```python
from build123d import *

# Parameters (mm, degrees)
CUT_EXTRUDE1_SOCKET_SLIT_DEPTH  = 18.588952107
CIRPATTERN1_PATTERN_SLITS_COUNT = 4
CHAMFER1_SIZE                   = 0.762
FILLET1_R                       = 0.762


with BuildPart() as part:
    # Sketch1 → Revolve1 - main body (revolve)
    with BuildSketch(Plane.XY):
        with BuildLine():
            Line((0, 0), (0, 13.751471687))
            ThreePointArc((0, 13.751471687), (-4.410161159, 16.183513693), (-4.70662, 21.211083874))
            Line((-4.70662, 21.211083874), (-6.08215434, 21.867194596))
            Line((-6.08215434, 21.867194596), (-7.191504241, 21.867194596))
            ThreePointArc((-7.191504241, 21.867194596), (-7.193470164, 16.069866844), (-3.175, 11.891241417))
            Line((-3.175, 11.891241417), (-3.175, 9.351241417))
            ThreePointArc((-3.175, 9.351241417), (-4.937771284, 3.538112772), (0, 0))
        make_face()
    revolve(axis=Axis((0, 0, 0), (0, -1, 0)))

    # Sketch2 → Cut-Extrude1 - socket slit (cut, through all)
    with BuildSketch(Plane(origin=(0, 13.751471687, 0), x_dir=(-1, 0, 0), z_dir=(0, -1, 0))):
        with BuildLine():
            Line((0, 0.254), (9.731504241, 0.254))
            ThreePointArc((9.731504241, 0.254), (9.985504241, 0), (9.731504241, -0.254))
            Line((9.731504241, -0.254), (0, -0.254))
            ThreePointArc((0, -0.254), (-0.254, 0), (0, 0.254))
        make_face()
    cut_extrude1_socket_slit = extrude(amount=-CUT_EXTRUDE1_SOCKET_SLIT_DEPTH, mode=Mode.SUBTRACT)

    # CirPattern1 - pattern slits: Cut-Extrude1 - socket slit ×4 about axis
    cirpattern1_pattern_slits_axis = Axis((0, 0, 0), (0, 1, 0))
    for i in range(1, CIRPATTERN1_PATTERN_SLITS_COUNT):
        add(cut_extrude1_socket_slit.rotate(cirpattern1_pattern_slits_axis, i * 360 / CIRPATTERN1_PATTERN_SLITS_COUNT), mode=Mode.SUBTRACT)

    # Chamfer1
    # the kernel refuses this chamfer: 0.762 mm, written as the material it takes off along each edge
    with BuildSketch(Plane(origin=(9.146639708, 21.867194596, 0.254), x_dir=(0, 0.02749587661058728, 0.9996219169112966), z_dir=(-1, 0, 0)), Plane(origin=(0.254, 21.867194596, -9.146639708), x_dir=(0.9996219169112966, 0.02749587661058728, 0), z_dir=(0, 0, 1)), Plane(origin=(-0.254, 21.867194596, 9.146639708), x_dir=(-0.9996219169112966, 0.027495876610587285, 0), z_dir=(0, 0, -1))) as chamfer1_piece_1:
        Polygon((CHAMFER1_SIZE * 0.999621916911, -CHAMFER1_SIZE * 0.0274958766106), (-CHAMFER1_SIZE * 0.0274958766106, -CHAMFER1_SIZE * 0.999621916911), (0, 0), align=None)
    extrude(amount=5.029413832, mode=Mode.SUBTRACT)
    with BuildSketch(Plane(origin=(4.117225876, 21.867194596, -0.254), x_dir=(0, -0.9996219169112968, 0.027495876610586327), z_dir=(1, 0, 0)), Plane(origin=(-0.254, 21.867194596, -4.117225876), x_dir=(0.027495876610586327, -0.9996219169112968, 0), z_dir=(0, 0, -1)), Plane(origin=(0.254, 21.867194596, 4.117225876), x_dir=(-0.027495876610586327, -0.9996219169112968, 0), z_dir=(0, 0, 1)), Plane(origin=(-9.146639708, 21.867194596, -0.254), x_dir=(0, -0.9996219169112968, 0.027495876610586327), z_dir=(1, 0, 0)), Plane(origin=(-4.117225876, 21.867194596, 0.254), x_dir=(0, -0.9996219169112968, -0.027495876610586327), z_dir=(-1, 0, 0))) as chamfer1_piece_2:
        Polygon((CHAMFER1_SIZE * 0.999621916911, CHAMFER1_SIZE * 0.0274958766106), (-CHAMFER1_SIZE * 0.0274958766106, CHAMFER1_SIZE * 0.999621916911), (0, 0), align=None)
    extrude(amount=5.029413832, mode=Mode.SUBTRACT)

    # Fillet1
    fillet1_edges = [part.edges().sort_by_distance(p)[0] for p in [
        (3.175, 11.891241417, 0),
        (3.175, 9.351241417, 0),
    ]]
    fillet(fillet1_edges, radius=FILLET1_R)


solid = part.part
```
Here's how the part is built. I have some questions about the finished solid (model axes, mm). A direction names the side the tool comes from. Coordinates: 2 decimals unless noted, no trailing zeros. Write each loop counter-clockwise with the first axis right and the second up, starting at its lowest first coordinate (ties: lowest second). Pieces come first, ordered by that corner, then holes. Notation, with made-up numbers: M -16,32.5 L 4,32.5 A12 cw 4,41.5 Z; hole C 37,-20 d9. An arc over 180 degrees is marked long. Answer as CSV lines item,"result". Start each with the question number.
Q1. If we mould it in two halves opening along Y, with no side actions, what happens to faces 1 (the flat face through (4.5, 21.867, -4.5)), 2 (the cylindrical face through (2.52, 10.55, 1.93)), 3 (the flat face through (-6, 17, 0.254))? For each: pulls with the +Y half, pulls with the -Y half, needs draft (parallel to the pull), parting line crosses it, or undercut.
Q2. Suppose I cut it at A-A, the plane z = -6.25. List the corners of the cut face in (x, y) for me.
Q3. Suppose I cut it at B-B, the plane y = 19.25. List the corners of the cut face in (x, z) for me.
Q4. Suppose I cut it at C-C, the plane x = 6.25. List the corners of the cut face in (y, z) for me, then the cut area to 3 significant figures.
Q5. Suppose I cut it at D-D, the plane y = 5.75. List the corners of the cut face in (x, z) for me.
Q6. Will these pins go through, and if not, where does the flat tip stop? pin 1 Ø6 at (y, z) = (16.5, -6) entering from +X; pin 2 Ø8 at (x, y) = (3.5, 17.5) entering from -Z; pin 3 Ø1.5 at (y, z) = (18, -5.5) entering from -X; pin 4 Ø3.5 at (y, z) = (18, -5.5) entering from -X.
Q7. For faces 4 (the flat face through (0.254, 17, -6)), 5 (the flat face through (6, 17, 0.254)), 6 (the conical face through (-3.64, 21.4, -3.57)), 7 (the flat face through (-4.5, 21.867, 4.5)), which set-ups out of +Z, -Z, +X, -X, +Y, -Y let a thin tool reach every point of the face, with its end or its side?
Q8. I need wall thicknesses on probe 1 along X at (y, z) = (5.5, -2.25); probe 2 along Z at (x, y) = (-6.25, 20.25); probe 3 along X at (y, z) = (11.25, 0) (3 decimals). Which ranges of each line are inside material? Lowest first, please. Write a range as [from, to].
Entries:
1,face 1,"pulls with the +Y half"
1,face 2,"undercut"
1,face 3,"needs draft"
2,outline,"M -3.56,21.87 A4.59 ccw -0.25,14.38 L -0.25,21.11 L -1.02,21.87 Z; M 0.25,14.38 A4.59 ccw 3.56,21.87 L 1.02,21.87 L 0.25,21.11 Z"
3,outline,"M -7.75,-0.25 A7.75 ccw -0.25,-7.75 L -0.25,-5.2 A5.21 cw -5.2,-0.25 Z; M -7.75,0.25 L -5.2,0.25 A5.21 cw -0.25,5.2 L -0.25,7.75 A7.75 ccw Z; M 0.25,-7.75 A7.75 ccw 7.75,-0.25 L 5.2,-0.25 A5.21 cw 0.25,-5.2 Z; M 0.25,5.2 A5.21 cw 5.2,0.25 L 7.75,0.25 A7.75 ccw 0.25,7.75 Z"
4,outline,"M 14.38,-0.25 A4.59 ccw 21.87,-3.56 L 21.87,-1.02 L 21.11,-0.25 Z; M 14.38,0.25 L 21.11,0.25 L 21.87,1.02 L 21.87,3.56 A4.59 ccw Z"
4,area,"53.5 mm²"
5,outline,"C 0,0 d10.37"
6,pin 1,"stops at x = 6.93"
6,pin 2,"stops at z = -7.75"
6,pin 3,"stops at x = -6.06"
6,pin 4,"stops at x = -6.74"
7,face 4,"+Z, -Z, +Y"
7,face 5,"+X, -X, +Y"
7,face 6,"+Y"
7,face 7,"+Z, -Z, +X, -X, +Y"
8,probe 1,"x = [-4.7, 4.7]"
8,probe 2,"z = [-4.41, -0.25], [0.25, 4.41]"
8,probe 3,"x = [-3.175, 3.175]"
